Geometry: final body of the model. Coordinates: model frame, mm. Face numbers are marked on the shaded views. A direction names the side the tool comes from. Give positions to 0.01 mm unless a question says otherwise; leave off trailing zeros. Write each loop counter-clockwise with the first axis right and the second up, starting at its lowest first coordinate (ties: lowest second). Pieces come first, ordered by that corner, then holes.
Autodesk Inventor part; units mm, degrees
ref_plane "XZ Plane" through (0, 0, 0) normal (0, 1, 0) x (-1, 0, 0)
ref_plane "XY Plane" through (0, 0, 0) normal (0, 0, 1) x (1, 0, 0)
sketch "Sketch1" plane through (0, 0, 0) normal (0, 0, 1) x (1, 0, 0)
  circle A0 centre (0, 0) radius 8
  dimension "d0" = 16
extrude "Extrusion1" add sketch "Sketch1" along normal blind 73
sketch "Sketch2" plane through (0, 0, 0) normal (0, 0, -1) x (-1, 0, 0)
  circle A0 centre (0, 0) radius 8
  circle A1 centre (0, 0) radius 5
  dimension "d6" = 10
extrude "Extrusion2" cut sketch "Sketch2" against normal blind 6.2
sketch "Sketch3" plane through (0, 0, 73) normal (0, 0, 1) x (1, 0, 0)
  circle A0 centre (0, 0) radius 8
  circle A1 centre (0, 0) radius 5
  dimension "d9" = 10
extrude "Extrusion3" cut sketch "Sketch3" against normal blind 6.2
chamfer "Chamfer2" distance 1 angle 45 2 edges at (-5, 0, 73) (5, 0, 0)
sketch "Sketch4" plane through (0, 0, 0) normal (0, 0, -1) x (-1, 0, 0)
  circle A0 centre (0, 0) radius 4
hole "Hole1" at (0, 0, 0) direction (0, 0, 1) diameter 4.917 depth 12 tip angle 118
sketch "Sketch5" plane through (0, 0, 73) normal (0, 0, 1) x (1, 0, 0)
  circle A0 centre (0, 0) radius 4
hole "Hole2" at (0, 0, 73) direction (0, 0, -1) diameter 4.917 depth 12 tip angle 118
chamfer "Chamfer3" distance 0.5 angle 45 2 edges at (0, 2.4585, 73) (0, -2.4585, 0)
sketch "Sketch6" plane through (0, 0, 66.8) normal (0, 0, 1) x (1, 0, 0)
  circle A0 centre (0, 0) radius 8
  circle A1 centre (0, 0) radius 6
  dimension "d32" = 12
extrude "Extrusion4" cut sketch "Sketch6" against normal blind 60.6
ref_plane "Work Plane1" through (6, 0, 66.8) normal (1, 0, 0) x (0, 1, 0)
sketch "Sketch7" plane through (6, 0, 66.8) normal (1, 0, 0) x (0, 1, 0)
  line L0 (-6, -60.6) -> (6, -60.6)
  line L1 (6, 0) -> (-6, 0)
  circle A0 centre (0, -30.3) radius 3
  point P0 (0, -66.8)
  dimension "d35" = 6
  dimension "d36" = 30.3
hole "Hole3" at (6, 0, 36.5) direction (-1, 0, 0) diameter 6 depth 4 tip angle 118
properties part number "EIXO DIANTEIRO(34)" material "Carbon Steel"
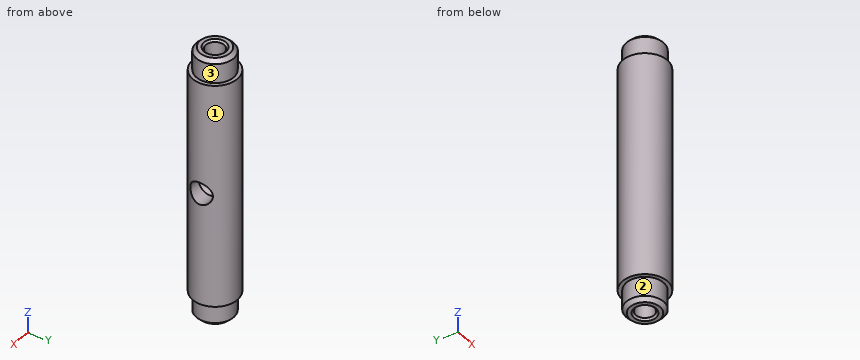
Q1. Access query for the marked faces 1, 2 and 3. Directions: +Z, -Z, +X, -X, +Y, -Y. A direction counts if a zero-diameter tool reaches every point of the face in a straight line with its end or side. Return the directions, or none.
Filled sheet:
face 1: +Z, -Z
face 2: -Z
face 3: +Z
Q2. Pin query (flat end, axial travel): P1, Ø5.5, axis at x = 0, y = 0, coming from the -Z side; P2, Ø4, axis at x = 0, y = 0, coming from the +Z side; P3, Ø6, axis at x = -4.5, y = -4.5, coming from the +Z side; P4, Ø1, axis at y = -1.5, z = 62, coming from the +X side. Return the tip coordinate at first contact, or that it passes through.
Filled sheet:
P1: stops at z = 0.21
P2: stops at z = 60.72
P3: stops at z = 73
P4: stops at x = 5.92
Q3. Section B-B on z = 18.5. Output: boundary loops of the cut face in (x, y).
Filled sheet:
outline: circle Ø12 at (0, 0)
Q4. Section A-A on z = 62. Output: boundary loops of the cut face in (x, y).
Filled sheet:
outline: circle Ø12 at (0, 0); hole circle Ø4.92 at (0, 0)
Q5. Ray query, line 1 along Z through (x, y) = (0.5, 5.5); line 2 along Y through (x, z) = (0, 63.5); line 3 along Z through (x, y) = (4.25, 1.5). Return the intervals inside material, ascending.
Filled sheet:
line 1: z = 6.2 to 66.8
line 2: y = -6 to -2.46, 2.46 to 6
line 3: z = 0.51 to 33.9, 39.1 to 72.49
